from build123d import *

# Parameters (mm, degrees)
EXTRUDE_1_DEPTH     = 3
SKETCH_3_R          = 1.5
CUT_EXTRUDE_1_DEPTH = 37.796738986
SKETCH_4_W          = 15
SKETCH_4_H          = 3
CUT_EXTRUDE_2_DEPTH = 39.742741271
FILLET_1_R          = 1.25


with BuildPart() as part:
    # ｽｹｯﾁ1 → ﾎﾞｽ - 押し出し1 (new, symmetric)
    with BuildSketch(Plane.XY):
        with BuildLine():
            Line((-15.25, -6), (-11.532562595, -6))
            ThreePointArc((-11.532562595, -6), (0, -13), (11.532562595, -6))
            Line((11.532562595, -6), (15.25, -6))
            ThreePointArc((15.25, -6), (16, -5.75), (16.75, -6))
            Line((16.75, -6), (36, -6))
            Line((36, -6), (36, -1))
            Line((36, -1), (7.937253933, -1))
            ThreePointArc((7.937253933, -1), (0, -8), (-7.937253933, -1))
            Line((-7.937253933, -1), (-21, -1))
            Line((-21, -1), (-21, -6))
            Line((-21, -6), (-16.75, -6))
            ThreePointArc((-16.75, -6), (-16, -5.75), (-15.25, -6))
        make_face()
    extrude(amount=EXTRUDE_1_DEPTH, both=True)

    # ｽｹｯﾁ3 → ｶｯﾄ - 押し出し1 (cut, through all)
    with BuildSketch(Plane.XZ.offset(6)):
        with Locations((-16, 0)):
            Circle(SKETCH_3_R)
        with Locations((16, 0)):
            Circle(SKETCH_3_R)
    extrude(amount=-CUT_EXTRUDE_1_DEPTH, mode=Mode.SUBTRACT)

    # ｽｹｯﾁ4 → ｶｯﾄ - 押し出し2 (cut, through all)
    with BuildSketch(Plane.XY.offset(3)):
        with Locations((28.5, -2.5)):
            Rectangle(SKETCH_4_W, SKETCH_4_H)
    extrude(amount=-CUT_EXTRUDE_2_DEPTH, mode=Mode.SUBTRACT)

    # ﾌｨﾚｯﾄ1
    fillet_1_edges = [part.edges().sort_by_distance(p)[0] for p in [
        (11.532562595, -6, 0),
        (-11.532562595, -6, 0),
        (21, -4, 0),
    ]]
    fillet(fillet_1_edges, radius=FILLET_1_R)


solid = part.part
Design review of the part built by this model. Coordinates are the model's own, in mm. A direction names the side the tool comes from. Give positions to 0.01 mm unless a question says otherwise; leave off trailing zeros. Write each loop counter-clockwise with the first axis right and the second up, starting at its lowest first coordinate (ties: lowest second). Pieces come first, ordered by that corner, then holes. Notation, with made-up numbers: M 42,26 L 97,26 A30 ccw 97,56 Z; hole C 56,75.25 d3. An arc over 180 degrees is marked long. Return JSON: item names as keys, results as strings. Group by question number.
Item 1: Clearance check with flat-ended pins moving along their axes: pin 1 Ø1.5 at (y, z) = (-10.5, 0.5) entering from +X; pin 2 Ø1.9 at (y, z) = (-2, -1) entering from +X; pin 3 Ø3.5 at (x, z) = (-19.5, 1) entering from -Y; pin 4 Ø2.5 at (x, z) = (16, 0) entering from -Y. State where each tip first meets the part, or that it passes through.
Item 2: Take a section at D-D (y = -2.25). Give the boundary of the cut face in (x, z).
Item 3: Wall thickness on line 1 along Z through (x, y) = (-16, -3.65); line 2 along X through (y, z) = (-3.1, 0); line 3 along X through (y, z) = (-4.8, 0): over which ranges is each line inside the solid? List them lowest first.
Item 4: Take a section at C-C (y = -7.25). Give the boundary of the cut face in (x, z).
Item 5: Take a section at A-A (x = -16). Give the boundary of the cut face in (y, z).
Item 6: Tool access review of faces 1 (the flat face through (21, -2, 0)), 2 (the flat face through (-14, -6, 0)), 3 (the flat face through (14, -6, 0)): name each direction out of +Z, -Z, +X, -X, +Y, -Y from which nothing blocks a thin tool from reaching the whole face with its end or side.
Item 7: The part is to be moulded in two halves that separate along Z. For faces 4 (the flat face through (29, -4, 0)), 5 (the flat face through (7, -6, 3)), 6 (the cylindrical face through (-17.5, -3.54, 0.07)), say which applies: pulls with the +Z half, pulls with the -Z half, needs draft (parallel to the pull), parting line crosses it, or undercut.
Item 8: Take a section at B-B (z = 0). Give the boundary of the cut face in (x, y), plus the area to 3 significant figures.
Return value:
{
 "1": {"pin 1": "stops at x = 8.6", "pin 2": "stops at x = 21.02", "pin 3": "stops at y = -6", "pin 4": "passes through"},
 "2": {"outline": "M -21,-3 L -7.68,-3 L -7.68,3 L -21,3 Z; M 7.68,-3 L 21,-3 L 21,3 L 7.68,3 Z; hole C -16,0 d3; hole C 16,0 d3"},
 "3": {"line 1": "z = -3 to -1.5, 1.5 to 3", "line 2": "x = -21 to -17.5, -14.5 to -7.37, 7.37 to 14.5, 17.5 to 21.05", "line 3": "x = -21 to -17.5, -14.5 to -6.4, 6.4 to 14.5, 17.5 to 36"},
 "4": {"outline": "M -10.79,-3 L -3.38,-3 L -3.38,3 L -10.79,3 Z; M 3.38,-3 L 10.79,-3 L 10.79,3 L 3.38,3 Z"},
 "5": {"outline": "M -5.75,-3 L -1,-3 L -1,-1.5 L -5.75,-1.5 Z; M -5.75,1.5 L -1,1.5 L -1,3 L -5.75,3 Z"},
 "6": {"face 1": "+Z, -Z, +X, +Y", "face 2": "+Z, -Z, -X, -Y", "face 3": "+Z, -Z, +X, -Y"},
 "7": {"face 4": "needs draft", "face 5": "pulls with the +Z half", "face 6": "undercut"},
 "8": {"outline": "M -21,-6 L -17.5,-6 L -17.5,-1 L -21,-1 Z; M -14.5,-6 L -12.27,-6 A1.25 cw -11.19,-6.61 A13 ccw 11.19,-6.61 A1.25 cw 12.27,-6 L 14.5,-6 L 14.5,-1 L 7.94,-1 A8 cw -7.94,-1 L -14.5,-1 Z; M 17.5,-6 L 36,-6 L 36,-4 L 22.25,-4 A1.25 cw 21,-2.75 L 21,-1 L 17.5,-1 Z", "area": "241 mm2"}
}
